Build history of the part. All positions in model axes, mm. Face numbers are marked on the shaded views. A direction names the side the tool comes from. Coordinates: 2 decimals unless noted, no trailing zeros. Loops run counter-clockwise (first coordinate to the right, second up) from the corner with the lowest first, then second, coordinate; pieces in that order, holes last.
Item 1: Cut at A-A (x = -3.5). List the corners of the cut face in (y, z), and give its area (3 significant figures).
Item 2: Mould opens along Z. For the marked faces 3, 4 and 5 say: released by +Z, released by -Z, zero draft, split by the parting line, or undercut.
Item 3: Cut at D-D (z = 0). List the corners of the cut face in (x, y).
Item 4: Cut at B-B (y = 31). List the corners of the cut face in (x, z), and give its area (3 significant figures).
Item 5: 3-axis set-ups, long thin cutter, end or side, ignore diameter. For the marked faces 1 and 2: which of +Z, -Z, +X, -X, +Y, -Y reach the whole face in a straight line?
Item 6: Drill centre lines: line 1 along Y through (x, z) = (-14.5, 3.3); line 2 along Z through (x, y) = (-4, 38.5); line 3 along Z through (x, y) = (-10, 41). Where is each one in solid material? Low to high.
Item 7: Flat gauge pins, fed straight in: pin 1 (4 mm diameter, centred on x = -14.5, y = 35, fed in from -Z); pin 2 (2 mm diameter, centred on y = 32.5, z = -4, fed in from -X); pin 3 (1.9 mm diameter, centred on x = -14.5, y = 10, fed in from -Z) (1 decimal); pin 4 (3 mm diameter, centred on y = 25.5, z = -1, fed in from -X). Where does each tip first touch, or does it go through?
Item 8: Cut at C-C (z = 3.5). List the corners of the cut face in (x, y), and give its area (3 significant figures).
from build123d import *

# Parameters (mm, degrees)
BOSS_EXTRUDE1_DEPTH                                 = 45
SKETCH2_R                                           = 1
CUT_EXTRUDE1_DEPTH                                  = 5
SKETCH3_R                                           = 2.5
CUT_EXTRUDE2_DEPTH                                  = 6
CSK_FOR_M2_COUNTERSUNK_FLAT_HEAD_SCREW1_D           = 2.4
CSK_FOR_M2_COUNTERSUNK_FLAT_HEAD_SCREW1_CSINK_D     = 4.4
CSK_FOR_M2_COUNTERSUNK_FLAT_HEAD_SCREW1_CSINK_ANGLE = 90


with BuildPart() as part:
    # Sketch1 → Boss-Extrude1 (new body)
    with BuildSketch(Plane(origin=(0, 0, 0), x_dir=(1, 0, 0), z_dir=(0, 1, 0))):
        with BuildLine():
            Line((0, 3), (-9, 3))
            Line((-9, 3), (-9, 5))
            Line((-9, 5), (0, 5))
            ThreePointArc((0, 5), (5, 0), (0, -5))
            Line((0, -5), (-18, -5))
            Line((-18, -5), (-18, -3))
            Line((-18, -3), (0, -3))
            ThreePointArc((0, -3), (3, 0), (0, 3))
        make_face()
    extrude(amount=BOSS_EXTRUDE1_DEPTH)

    # Sketch2 → Cut-Extrude1 (cut)
    with BuildSketch(Plane(origin=(0, 0, -5), x_dir=(-1, 0, 0), z_dir=(0, 0, -1))):
        with Locations((9, 17.5)):
            Circle(SKETCH2_R)
    extrude(amount=-CUT_EXTRUDE1_DEPTH, mode=Mode.SUBTRACT)

    # Sketch3 → Cut-Extrude2 (cut)
    with BuildSketch(Plane(origin=(0, 0, 0), x_dir=(0, 0, -1), z_dir=(1, 0, 0))):
        Circle(SKETCH3_R)
    extrude(amount=CUT_EXTRUDE2_DEPTH, mode=Mode.SUBTRACT)

    # CSK for M2 Countersunk Flat Head Screw1 (through all)
    with Locations(Plane(origin=(-14.5, 35, 5), x_dir=(1, 0, 0), z_dir=(0, 0, 1))):
        with Locations((0, 0), (0, -25)):
            CounterSinkHole(CSK_FOR_M2_COUNTERSUNK_FLAT_HEAD_SCREW1_D / 2, CSK_FOR_M2_COUNTERSUNK_FLAT_HEAD_SCREW1_CSINK_D / 2, counter_sink_angle=CSK_FOR_M2_COUNTERSUNK_FLAT_HEAD_SCREW1_CSINK_ANGLE)


solid = part.part
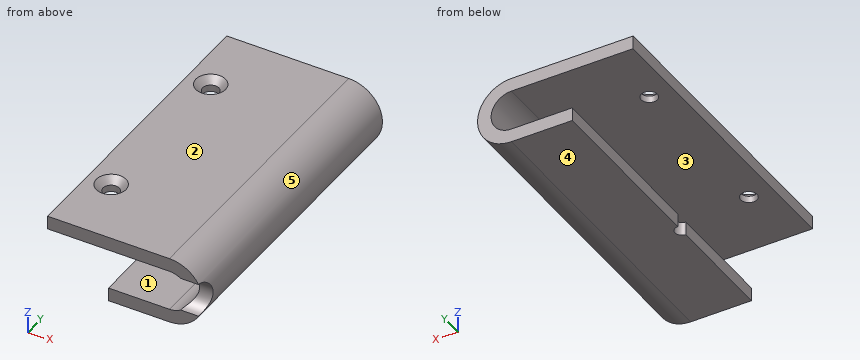
Filled sheet:
1. outline: (0, -5) - (45, -5) - (45, -3) - (0, -3) - close; (0, 3) - (45, 3) - (45, 5) - (0, 5) - close
1. area: 180 mm2
2. face 3: undercut
2. face 4: released by -Z
2. face 5: split by the parting line
3. outline: (3, 2.5) - (5, 2.5) - (5, 45) - (3, 45) - close
4. outline: (-18, 3) - (0, 3) arc R3 cw to (0, -3) - (-9, -3) - (-9, -5) - (0, -5) arc R5 ccw to (0, 5) - (-18, 5) - close
4. area: 79.1 mm2
5. face 1: -X, +Y, -Y
5. face 2: +Z, +X, -X, +Y, -Y
6. line 1: y = 0 to 8.8, 11.2 to 33.8, 36.2 to 45
6. line 2: z = -5 to -3, 3 to 5
6. line 3: z = 3 to 5
7. pin 1: stops at z = 3
7. pin 2: stops at x = -9
7. pin 3: passes through
7. pin 4: stops at x = 1.66
8. outline: (-18, 0) - (3.57, 0) - (3.57, 45) - (-18, 45) - close; hole circle Ø2.4 at (-14.5, 10); hole circle Ø2.4 at (-14.5, 35)
8. area: 962 mm2
